Part model, mm, in its own coordinate system. Round coordinates to 2 decimals unless told otherwise and drop trailing zeros. Use CSV: the item, a comma, the result in double quotes.
```python
from build123d import *

# Parameters (mm, degrees)
SKETCH1_R           = 2.1
BOSS_EXTRUDE1_DEPTH = 750


with BuildPart() as part:
    # Sketch1 → Boss-Extrude1 (new body)
    with BuildSketch(Plane.XY.offset(10)):
        with BuildLine():
            Line((-12.84, -8.2), (-15.499339828, -8.2))
            Line((-15.499339828, -8.2), (-15.499339828, -6.56))
            Line((-15.499339828, -6.56), (-12.84, -3.900660172))
            Line((-12.84, -3.900660172), (-7.16, -3.900660172))
            Line((-7.16, -3.900660172), (-4.500660172, -6.56))
            Line((-4.500660172, -6.56), (-4.500660172, -8.2))
            Line((-4.500660172, -8.2), (-7.16, -8.2))
            Line((-7.16, -8.2), (-5.36, -10))
            Line((-5.36, -10), (5.36, -10))
            Line((5.36, -10), (7.16, -8.2))
            Line((7.16, -8.2), (4.500660172, -8.2))
            Line((4.500660172, -8.2), (4.500660172, -6.56))
            Line((4.500660172, -6.56), (7.16, -3.900660172))
            Line((7.16, -3.900660172), (12.84, -3.900660172))
            Line((12.84, -3.900660172), (15.499339828, -6.56))
            Line((15.499339828, -6.56), (15.499339828, -8.2))
            Line((15.499339828, -8.2), (12.84, -8.2))
            Line((12.84, -8.2), (14.64, -10))
            Line((14.64, -10), (18.2, -10))
            ThreePointArc((18.2, -10), (19.472792206, -9.472792206), (20, -8.2))
            Line((20, -8.2), (20, -4.64))
            Line((20, -4.64), (18.2, -2.84))
            Line((18.2, -2.84), (18.2, -5.499339828))
            Line((18.2, -5.499339828), (16.56, -5.499339828))
            Line((16.56, -5.499339828), (13.900660172, -2.84))
            Line((13.900660172, -2.84), (13.900660172, 2.84))
            Line((13.900660172, 2.84), (16.56, 5.499339828))
            Line((16.56, 5.499339828), (18.2, 5.499339828))
            Line((18.2, 5.499339828), (18.2, 2.84))
            Line((18.2, 2.84), (20, 4.64))
            Line((20, 4.64), (20, 8.2))
            ThreePointArc((20, 8.2), (19.472792206, 9.472792206), (18.2, 10))
            Line((18.2, 10), (14.64, 10))
            Line((14.64, 10), (12.84, 8.2))
            Line((12.84, 8.2), (15.499339828, 8.2))
            Line((15.499339828, 8.2), (15.499339828, 6.56))
            Line((15.499339828, 6.56), (12.84, 3.900660172))
            Line((12.84, 3.900660172), (7.16, 3.900660172))
            Line((7.16, 3.900660172), (4.500660172, 6.56))
            Line((4.500660172, 6.56), (4.500660172, 8.2))
            Line((4.500660172, 8.2), (7.16, 8.2))
            Line((7.16, 8.2), (5.36, 10))
            Line((5.36, 10), (-5.36, 10))
            Line((-5.36, 10), (-7.16, 8.2))
            Line((-7.16, 8.2), (-4.500660172, 8.2))
            Line((-4.500660172, 8.2), (-4.500660172, 6.56))
            Line((-4.500660172, 6.56), (-7.16, 3.900660172))
            Line((-7.16, 3.900660172), (-12.84, 3.900660172))
            Line((-12.84, 3.900660172), (-15.499339828, 6.56))
            Line((-15.499339828, 6.56), (-15.499339828, 8.2))
            Line((-15.499339828, 8.2), (-12.84, 8.2))
            Line((-12.84, 8.2), (-14.64, 10))
            Line((-14.64, 10), (-25.36, 10))
            Line((-25.36, 10), (-27.16, 8.2))
            Line((-27.16, 8.2), (-24.500660172, 8.2))
            Line((-24.500660172, 8.2), (-24.500660172, 6.56))
            Line((-24.500660172, 6.56), (-27.16, 3.900660172))
            Line((-27.16, 3.900660172), (-32.84, 3.900660172))
            Line((-32.84, 3.900660172), (-35.499339828, 6.56))
            Line((-35.499339828, 6.56), (-35.499339828, 8.2))
            Line((-35.499339828, 8.2), (-32.84, 8.2))
            Line((-32.84, 8.2), (-34.64, 10))
            Line((-34.64, 10), (-38.2, 10))
            ThreePointArc((-38.2, 10), (-39.472792206, 9.472792206), (-40, 8.2))
            Line((-40, 8.2), (-40, 4.64))
            Line((-40, 4.64), (-38.2, 2.84))
            Line((-38.2, 2.84), (-38.2, 5.499339828))
            Line((-38.2, 5.499339828), (-36.56, 5.499339828))
            Line((-36.56, 5.499339828), (-33.900660172, 2.84))
            Line((-33.900660172, 2.84), (-33.900660172, -2.84))
            Line((-33.900660172, -2.84), (-36.56, -5.499339828))
            Line((-36.56, -5.499339828), (-38.2, -5.499339828))
            Line((-38.2, -5.499339828), (-38.2, -2.84))
            Line((-38.2, -2.84), (-40, -4.64))
            Line((-40, -4.64), (-40, -8.2))
            ThreePointArc((-40, -8.2), (-39.472792206, -9.472792206), (-38.2, -10))
            Line((-38.2, -10), (-34.64, -10))
            Line((-34.64, -10), (-32.84, -8.2))
            Line((-32.84, -8.2), (-35.499339828, -8.2))
            Line((-35.499339828, -8.2), (-35.499339828, -6.56))
            Line((-35.499339828, -6.56), (-32.84, -3.900660172))
            Line((-32.84, -3.900660172), (-27.16, -3.900660172))
            Line((-27.16, -3.900660172), (-24.500660172, -6.56))
            Line((-24.500660172, -6.56), (-24.500660172, -8.2))
            Line((-24.500660172, -8.2), (-27.16, -8.2))
            Line((-27.16, -8.2), (-25.36, -10))
            Line((-25.36, -10), (-14.64, -10))
            Line((-14.64, -10), (-12.84, -8.2))
        make_face()
        with Locations(Location((-10, 0, 0), (0, 0, 180))):
            Circle(SKETCH1_R, mode=Mode.SUBTRACT)
        with Locations(Location((-30, 0, 0), (0, 0, 180))):
            Circle(SKETCH1_R, mode=Mode.SUBTRACT)
        with Locations(Location((10, 0, 0), (0, 0, 180))):
            Circle(SKETCH1_R, mode=Mode.SUBTRACT)
        Polygon((-13.900660172, 2.84), (-13.900660172, -2.84), (-17.300660172, -6.24), (-17.300660172, -8.2), (-22.699339828, -8.2), (-22.699339828, -6.24), (-26.099339828, -2.84), (-26.099339828, 2.84), (-22.699339828, 6.24), (-22.699339828, 8.2), (-17.300660172, 8.2), (-17.300660172, 6.24), align=None, mode=Mode.SUBTRACT)
        Polygon((-6.099339828, -2.84), (-6.099339828, 2.84), (-2.699339828, 6.24), (-2.699339828, 8.2), (2.699339828, 8.2), (2.699339828, 6.24), (6.099339828, 2.84), (6.099339828, -2.84), (2.699339828, -6.24), (2.699339828, -8.2), (-2.699339828, -8.2), (-2.699339828, -6.24), align=None, mode=Mode.SUBTRACT)
    extrude(amount=-BOSS_EXTRUDE1_DEPTH)


solid = part.part
```
(1) Drop flat-ended pins along their axis: P1, Ø2, axis at y = 4.5, z = -222.5, coming from the +X side; P2, Ø1.5, axis at x = 10.5, z = -139.5, coming from the -Y side; P3, Ø3, axis at x = 8.5, z = -263, coming from the +Y side; P4, Ø6, axis at x = -29.5, z = -221, coming from the +Y side. Give the stop position or say it passes through.
Reply:
P1,"x = 20"
P2,"y = -3.9"
P3,"y = 8.36"
P4,"y = 8.86"
(2) Probe probe 1 along X at (y, z) = (8, -329); probe 2 along X at (y, z) = (-2.75, -389); probe 3 along X at (y, z) = (6.5, -496). List the from-to ranges inside material, lowest first. Write a range as [from, to].
Reply:
probe 1,"[-40, -35.5], [-24.5, -22.7], [-17.3, -15.5], [-4.5, -2.7], [2.7, 4.5], [15.5, 20]"
probe 2,"[-33.9, -26.1], [-13.9, -6.1], [6.1, 13.9]"
probe 3,"[-40, -35.44], [-24.56, -22.7], [-17.3, -15.44], [-4.56, -2.7], [2.7, 4.56], [15.44, 20]"
(3) Cut at A-A, the plane z = -186. State how many separate pieces and enclosed holes the cut face has, then the cut area to 3 significant figures.
Reply:
separate pieces,"1"
enclosed holes,"5"
area,"426 mm2"
